Solid Edge part; units mm, degrees
sketch "Sketch1" plane through (0, 0, 0) normal (0, 0, 1) x (1, 0, 0)
  circle A0 centre (0, 0) radius 4.825
extrude "Protrusion1" add sketch "Sketch1" along normal blind 6.5
sketch "Sketch2" plane through (0, 0, 0) normal (0, 0, -1) x (1, 0, 0)
  line L0 (-6.8, 6.975) -> (6.8, 6.975)
  line L1 (6.8, 6.975) -> (6.8, -13.525)
  line L2 (6.8, -13.525) -> (-6.8, -13.525)
  line L3 (-6.8, -13.525) -> (-6.8, 6.975)
  dimension "D1" = 6.8
extrude "base" add sketch "Sketch2" along normal blind 1.6
sketch "Sketch3" plane through (0, 3.275, 0) normal (0, 0, 1) x (0, 1, 0)
  circle A0 centre (9.35, 2.6) radius 0.5
  circle A1 centre (9.35, 0) radius 0.5
  circle A2 centre (9.35, -2.6) radius 0.5
  dimension "D1" = 9.35
extrude "Cutout1" cut sketch "Sketch3" against normal through all
sketch "Sketch4" plane through (0, 3.275, 0) normal (0, 0, 1) x (-1, 0, 0)
  circle A0 centre (5, 8.2) radius 1.3
  circle A1 centre (-5, 8.2) radius 1.3
  dimension "D1" = 5
extrude "Cutout2" cut sketch "Sketch4" against normal through all
sketch "Sketch5" plane through (0, 3.275, -1.6) normal (0, 0, -1) x (1, 0, 0)
  line L0 (-6.8, 6.25) -> (6.8, 6.25)
  line L1 (6.8, 6.25) -> (6.8, -7.75)
  line L2 (6.8, -7.75) -> (-6.8, -7.75)
  line L3 (-6.8, -7.75) -> (-6.8, 6.25)
extrude "Extrusionsausprägung_3" add sketch "Sketch5" along normal blind 1.2
Geometry: final body of the model. Coordinates: model frame, mm. A direction names the side the tool comes from. Round coordinates to 2 decimals unless told otherwise and drop trailing zeros. Write each loop counter-clockwise with the first axis right and the second up, starting at its lowest first coordinate (ties: lowest second). Pieces come first, ordered by that corner, then holes.
Item 1: Section query B-B (z = -1.25). Return loops of the section in (x, y) (3 decimals), plus the area to 3 significant figures.
Item 2: Mould query, pull axis Y, two halves, no side actions, for faces 6 (the face through (0.192, 13.087, -0.789)), 7 (the face through (0, -6.975, -1)), 8 (the face through (-0.1, 11.7, -1.6)). Classes: +Y half, -Y half, draft (parallel to the pull), parting line (faces both ways), or undercut.
Item 3: Set-up query: faces 1 (the face through (0, -5, -1.6)), 2 (the face through (0, 11.025, -2)), 3 (the face through (-6.24, -5.32, -0.79)), 4 (the face through (4.6, -1.45, 3.2)), 5 (the face through (0, 4, -2.8)). Return all of +Z, -Z, +X, -X, +Y, -Y with unobstructed straight access to the full face (end or side cutting, diameter ignored); none if empty.
Item 4: Pin query (flat end, axial travel): P1, Ø0.8, axis at x = -0.5, y = 12, coming from the -Z side; P2, Ø1.5, axis at x = 0, y = 9.5, coming from the +Z side; P3, Ø0.6, axis at x = 1, z = -2, coming from the +Y side (3 decimals). Return the tip coordinate at first contact, or that it passes through.
Item 5: Material intervals for L1, parallel to Y at x = -2.6, z = -1.2 (3 decimals); L2, parallel to Y at x = 5, z = -0.95 (3 decimals); L3, parallel to Z at x = -2.25, y = -6, sorted ascending.
Item 6: Section query C-C (y = 0). Return loops of the section in (x, z) (3 decimals).
Item 7: Section query D-D (x = -2.6). Return loops of the section in (y, z) (3 decimals).
Item 8: Section query A-A (x = 0). Return loops of the section in (y, z) (3 decimals).
Completed:
1. outline: (-6.8, -6.975) - (6.8, -6.975) - (6.8, 13.525) - (-6.8, 13.525) - close; hole circle Ø2.6 at (-5, -4.925); hole circle Ø1 at (-2.6, 12.625); hole circle Ø1 at (0, 12.625); hole circle Ø1 at (2.6, 12.625); hole circle Ø2.6 at (5, -4.925)
1. area: 266 mm2
2. face 6: undercut
2. face 7: -Y half
2. face 8: draft
3. face 1: -Z, +X, -X, -Y
3. face 2: -Z, +X, -X, +Y
3. face 3: +Z, -Z
3. face 4: +Z
3. face 5: -Z, +X, -X, +Y, -Y
4. P1: stops at z = -1.6
4. P2: stops at z = 0
4. P3: stops at y = 11.025
5. L1: y = -6.975 to 12.125, 13.125 to 13.525
5. L2: y = -6.975 to -6.225, -3.625 to 13.525
5. L3: z = -1.6 to 0
6. outline: (-6.8, -2.8) - (6.8, -2.8) - (6.8, 0) - (4.825, 0) - (4.825, 6.5) - (-4.825, 6.5) - (-4.825, 0) - (-6.8, 0) - close
7. outline: (-6.975, -1.6) - (-2.975, -1.6) - (-2.975, -2.8) - (11.025, -2.8) - (11.025, -1.6) - (12.125, -1.6) - (12.125, 0) - (4.065, 0) - (4.065, 6.5) - (-4.065, 6.5) - (-4.065, 0) - (-6.975, 0) - close; (13.125, -1.6) - (13.525, -1.6) - (13.525, 0) - (13.125, 0) - close
8. outline: (-6.975, -1.6) - (-2.975, -1.6) - (-2.975, -2.8) - (11.025, -2.8) - (11.025, -1.6) - (12.125, -1.6) - (12.125, 0) - (4.825, 0) - (4.825, 6.5) - (-4.825, 6.5) - (-4.825, 0) - (-6.975, 0) - close; (13.125, -1.6) - (13.525, -1.6) - (13.525, 0) - (13.125, 0) - close
